The model under review builds one solid part; all positions refer to its coordinate system, in mm. Face numbers are marked on the shaded views. A direction names the side the tool comes from. Round coordinates to 2 decimals unless told otherwise and drop trailing zeros. Write each loop counter-clockwise with the first axis right and the second up, starting at its lowest first coordinate (ties: lowest second). Pieces come first, ordered by that corner, then holes.
Item 1: Clearance check with flat-ended pins moving along their axes: pin 1 Ø3 at (x, z) = (47, -23.5) entering from -Y; pin 2 Ø10 at (x, z) = (50.5, 23) entering from +Y; pin 3 Ø3 at (x, y) = (83.5, 5.5) entering from +Z; pin 4 Ø2 at (y, z) = (6.5, -3) entering from -X. State where each tip first meets the part, or that it passes through.
Item 2: Add section C-C (z = 7). Give the boundary of the cut face in (x, y) (1 decimal).
Item 3: Machinability: for the marked faces 4, 5 and 6, which of the approach directions +Z, -Z, +X, -X, +Y, -Y give a long, thin tool a straight path to every point of the face, cutting with its end or side? Answer none if there is none.
Item 4: To check wall thickness, follow L1, parallel to X at y = 5.5, z = 0; L2, parallel to Z at x = 0, y = 7; L3, parallel to X at y = 9, z = 8.5. State the ranges of each line that lie inside material, in increasing order.
Item 5: Add section D-D (z = 0). Give the boundary of the cut face in (x, y).
Item 6: Draft analysis for pull direction X (two halves, no side actions). For the marked faces 1, 2 and 3, state which applies: +X half, -X half, draft (parallel to the pull), parting line (faces both ways), or undercut.
Item 7: Add section B-B (y = 2). Give the boundary of the cut face in (x, z), plus the area to 3 significant figures.
Item 8: Add section A-A (x = 48). Give the boundary of the cut face in (y, z).
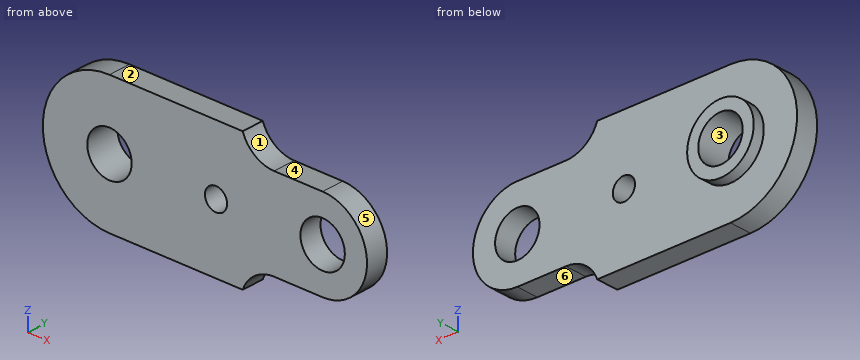
Autodesk Inventor part; units mm, degrees
ref_plane "YZ Plane" through (0, 0, 0) normal (1, 0, 0) x (0, 1, 0)
ref_plane "XZ Plane" through (0, 0, 0) normal (0, 1, 0) x (-1, 0, 0)
ref_plane "XY Plane" through (0, 0, 0) normal (0, 0, 1) x (1, 0, 0)
sketch "Sketch1" plane through (0, 0, 0) normal (0, 1, 0) x (-1, 0, 0)
  arc A0 (0, -30) -> (0, 30) centre (0, 0) ccw
  line L0 (0, -30) -> (-60, -30)
  arc A1 (-60, -30) -> (-74.1421, -20) centre (-74.1421, -35) ccw
  line L1 (-74.1421, -20) -> (-96, -20)
  line L2 (0, 0) -> (-48, 0)
  line L3 (-48, 0) -> (-96, 0)
  line L4 (0, 30) -> (-60, 30)
  arc A2 (-74.1421, 20) -> (-60, 30) centre (-74.1421, 35) ccw
  line L5 (-74.1421, 20) -> (-96, 20)
  arc A3 (-96, 20) -> (-96, -20) centre (-96, 0) ccw
  dimension "d1" = 30
  dimension "d2" = 48
  dimension "d3" = 60
  dimension "d4" = 15
  dimension "d5" = 20
  dimension "d6" = 96
extrude "Extrusion1" add sketch "Sketch1" along normal blind 10
hole "Hole2" at (0, 0, 0) at (96, 0, 0) direction (0, 1, 0) diameter 20 end through all
hole "Hole3" at (48, 0, 0) at (0, 0, 0) direction (0, 1, 0) diameter 10 end through all
sketch "Sketch3" plane through (0, 10, 0) normal (0, 1, 0) x (1, 0, 0)
  circle A0 centre (0, 0) radius 15
  dimension "d30" = 30
emboss "Emboss1" sketch "Sketch3" operation add depth 5 direction (0, -1, 0)
properties part number "SwivelBase"
Numbers:
1. pin 1: stops at y = 0
1. pin 2: stops at y = 10
1. pin 3: stops at z = 20
1. pin 4: stops at x = -29.93
2. outline: (-29.2, 0) - (-7.1, 0) - (-7.1, 15) - (-13.3, 15) - (-13.3, 10) - (-29.2, 10) - close; (7.1, 0) - (88.9, 0) - (88.9, 10) - (13.3, 10) - (13.3, 15) - (7.1, 15) - close; (103.1, 0) - (114.7, 0) - (114.7, 10) - (103.1, 10) - close
3. face 4: +Z, +X, +Y, -Y
3. face 5: +X, +Y, -Y
3. face 6: -Z, +X, +Y, -Y
4. L1: x = -30 to -10, 10 to 43, 53 to 86, 106 to 116
4. L2: z = -30 to -10, 10 to 30
4. L3: x = -28.77 to -5.27, 5.27 to 90.73, 101.27 to 114.1
5. outline: (-30, 0) - (-10, 0) - (-10, 15) - (-15, 15) - (-15, 10) - (-30, 10) - close; (10, 0) - (43, 0) - (43, 10) - (15, 10) - (15, 15) - (10, 15) - close; (53, 0) - (86, 0) - (86, 10) - (53, 10) - close; (106, 0) - (116, 0) - (116, 10) - (106, 10) - close
6. face 1: +X half
6. face 2: draft
6. face 3: undercut
7. outline: (0, -30) - (60, -30) arc R15 cw to (74.14, -20) - (96, -20) arc R20 ccw to (96, 20) - (74.14, 20) arc R15 cw to (60, 30) - (0, 30) arc R30 ccw to start; hole circle Ø20 at (0, 0); hole circle Ø10 at (48, 0); hole circle Ø20 at (96, 0)
7. area: 6,450 mm2
8. outline: (0, -30) - (10, -30) - (10, -5) - (0, -5) - close; (0, 5) - (10, 5) - (10, 30) - (0, 30) - close
